Work out the finished part from the listing and answer in its coordinate system (mm). A direction names the side the tool comes from. Round coordinates to 2 decimals unless told otherwise and drop trailing zeros. Order: outer loops, then holes, each group sorted by start corner. A loop starts at its lowest first (then second) coordinate and runs counter-clockwise, first axis right, second up.
from build123d import *

# Parameters (mm, degrees)
F0_R     = 7.1501
F1_DEPTH = 25.4


with BuildPart() as f1:
    # F0 (on Front) → F1 (new body)
    with BuildSketch(Plane.XZ):
        with BuildLine():
            ThreePointArc((12.951258, -13.970234), (17.458865, -7.621714), (19.05, 0))
            ThreePointArc((19.05, 0), (-7.799478, 17.380179), (-12.663453, -14.231636))
            ThreePointArc((-12.663453, -14.231636), (0.194398, -19.049008), (12.951258, -13.970234))
        make_face()
        Circle(F0_R, mode=Mode.SUBTRACT)
        with BuildLine():
            ThreePointArc((12.951258, -13.970234), (0.194398, -19.049008), (-12.663453, -14.231636))
            Line((-12.663453, -14.231636), (-12.663453, -19.05))
            Line((-12.663453, -19.05), (-12.663453, -67.058742))
            Line((-12.663453, -67.058742), (12.951258, -67.058742))
            Line((12.951258, -67.058742), (12.951258, -13.970234))
        make_face()
    extrude(amount=F1_DEPTH)


solid = f1.part
Item 1: Given pin 1 (11.5 mm diameter, centred on x = 0, z = 0, fed in from -Y); pin 2 (8 mm diameter, centred on y = -18, z = -9.5, fed in from +X); pin 3 (4 mm diameter, centred on y = -22, z = -8.5, fed in from -X); pin 4 (7.5 mm diameter, centred on y = -17.5, z = -33, fed in from -X), each flat-ended and moving along its own axis, determine where each tip first touches the part or whether it passes through.
Item 2: Find section D-D (z = -24.5). Write down the section's boundary in (x, y), plus the area to 3 significant figures.
Item 3: Find the intervals of material crossed by line 1 along Z through (x, y) = (0.5, -10.25); line 2 along X through (y, z) = (-16, -26); line 3 along X through (y, z) = (-14.25, -3), in increasing order.
Item 4: Find section C-C (y = -12.75). Write down the section's boundary in (x, z).
Item 5: A tool of negligible diameter and unlimited length cuts with its end or side. For faces 1 (the face through (0, -13, -67.059)), 2 (the face through (-12.663, -13, -40)), from which of +Z, -Z, +X, -X, +Y, -Y can it reach the whole face along a straight path? Write none if from no direction.
Item 6: Find section A-A (x = 0). Write down the section's boundary in (y, z).
Item 7: For a pull along X with two mould halves and no side action, classify faces 3 (the face through (12.951, -13, -41)), 4 (the face through (-1.55, -12.52, -6.98)), 5 (the face through (0, 0, -23)) as released by +X, released by -X, zero draft, split by the parting line, or undercut.
Item 8: Find section B-B (z = -3.5). Write down the section's boundary in (x, y), plus the area to 3 significant figures.
Model answer:
1. pin 1: passes through
1. pin 2: stops at x = 18.24
1. pin 3: stops at x = -17.91
1. pin 4: stops at x = -12.66
2. outline: (-12.66, -25.4) - (12.95, -25.4) - (12.95, 0) - (-12.66, 0) - close
2. area: 651 mm2
3. line 1: z = -67.06 to -7.13, 7.13 to 19.04
3. line 2: x = -12.66 to 12.95
3. line 3: x = -18.81 to -6.49, 6.49 to 18.81
4. outline: (-12.66, -67.06) - (12.95, -67.06) - (12.95, -13.97) arc R19.05 ccw to (19.05, 0) arc R19.05 ccw (long way) to (-12.66, -14.23) - close; hole circle Ø14.3 at (0, 0)
5. face 1: -Z, +X, -X, +Y, -Y
5. face 2: -Z, -X, +Y, -Y
6. outline: (-25.4, -67.06) - (0, -67.06) - (0, -7.15) - (-25.4, -7.15) - close; (-25.4, 7.15) - (0, 7.15) - (0, 19.05) - (-25.4, 19.05) - close
7. face 3: released by +X
7. face 4: undercut
7. face 5: zero draft
8. outline: (-18.73, -25.4) - (-6.23, -25.4) - (-6.23, 0) - (-18.73, 0) - close; (6.23, -25.4) - (18.73, -25.4) - (18.73, 0) - (6.23, 0) - close
8. area: 635 mm2
